Geometry: final body of the model. Coordinates: model frame, mm. A direction names the side the tool comes from. Give positions to 0.01 mm unless a question says otherwise; leave off trailing zeros. Loops run counter-clockwise (first coordinate to the right, second up) from the corner with the lowest first, then second, coordinate; pieces in that order, holes last. Notation, with made-up numbers: (-35, 34) - (-29, 34) arc R19 ccw to (-29, 69) - close; hole circle Ø6 at (55.25, 19). An arc over 180 degrees is marked (long way). Use one line per item in the form item = value.
```python
from build123d import *

# Parameters (mm, degrees)
BASE_FLANGE1_DEPTH = 212.725
FILLET1_R          = 6.35
SKETCH3_R          = 5.5626
SKETCH3_R_2        = 2.1082
CUT_EXTRUDE1_DEPTH = 7.62
CUT_EXTRUDE2_DEPTH = 246.533701925


# Read off the part's stored shape, not the designer's step: Base-Flange1
with BuildPart() as part:
    # Base-Flange1 outline → Base-Flange1 (new body)
    with BuildSketch(Plane.XY):
        with BuildLine():
            Line((-78.007365806, 1.016), (-95.25, 1.016))
            Line((-95.25, 1.016), (-95.25, 0))
            Line((-95.25, 0), (-78.007365806, 0))
            ThreePointArc((-78.007365806, 0), (-76.729452957, 0.520576705), (-76.17906817, 1.7859375))
            ThreePointArc((-76.17906817, 1.7859375), (0, 76.2), (76.17906817, 1.7859375))
            ThreePointArc((76.17906817, 1.7859375), (76.729452957, 0.520576705), (78.007365806, 0))
            Line((78.007365806, 0), (95.25, 0))
            Line((95.25, 0), (95.25, 1.016))
            Line((95.25, 1.016), (78.007365806, 1.016))
            ThreePointArc((78.007365806, 1.016), (77.43940454, 1.247367424), (77.194789079, 1.80975))
            ThreePointArc((77.194789079, 1.80975), (0, 77.216), (-77.194789079, 1.80975))
            ThreePointArc((-77.194789079, 1.80975), (-77.43940454, 1.247367424), (-78.007365806, 1.016))
        make_face()
    extrude(amount=BASE_FLANGE1_DEPTH)

    # Fillet1
    fillet1_edges = [part.edges().sort_by_distance(p)[0] for p in [
        (95.25, 0.508, 0),
        (-95.25, 0.508, 0),
        (95.25, 0.508, 212.725),
        (-95.25, 0.508, 212.725),
    ]]
    fillet(fillet1_edges, radius=FILLET1_R)

    # Sketch3 → Cut-Extrude1 (cut)
    with BuildSketch(Plane.XZ):
        with Locations((-85.725, 9.525)):
            Circle(SKETCH3_R)
        with Locations((-85.725, 25.4)):
            Circle(SKETCH3_R_2)
        with Locations((-85.725, 106.3752)):
            Circle(SKETCH3_R_2)
        with Locations((-85.725, 187.3504)):
            Circle(SKETCH3_R_2)
        with Locations((85.725, 9.525)):
            Circle(SKETCH3_R)
        with Locations((85.725, 25.4)):
            Circle(SKETCH3_R_2)
        with Locations((85.725, 106.3752)):
            Circle(SKETCH3_R_2)
        with Locations((85.725, 187.3504)):
            Circle(SKETCH3_R_2)
    extrude(amount=-CUT_EXTRUDE1_DEPTH, mode=Mode.SUBTRACT)

    # Sketch4 → Cut-Extrude2 (cut, through all)
    with BuildSketch(Plane(origin=(0, 0, 0), x_dir=(0, 0, -1), z_dir=(1, 0, 0))):
        with BuildLine():
            Line((-82.5627, -6.3754), (-82.5627, 9.525))
            ThreePointArc((-82.5627, 9.525), (-74.6125, 17.4752), (-66.6623, 9.525))
            Line((-66.6623, 9.525), (-66.6623, -6.3754))
            Line((-66.6623, -6.3754), (-82.5627, -6.3754))
        make_face()
    extrude(amount=CUT_EXTRUDE2_DEPTH, mode=Mode.SUBTRACT)


solid = part.part
```
(1) Cut plane D-D (x = 0). Return the cut outline in (y, z) (3 decimals), plus the area to 3 significant figures.
Solution:
outline = (76.2, 0) - (77.216, 0) - (77.216, 212.725) - (76.2, 212.725) - close
area = 216 mm2
(2) Pin query (flat end, axial travel): P1, Ø1, axis at x = -20, z = 180.5, coming from the +Y side; P2, Ø7.5, axis at x = 90, y = 7, coming from the -Z side; P3, Ø19, axis at x = 90.5, z = 135.5, coming from the +Y side; P4, Ø3, axis at y = 56.5, z = 132, coming from the +X side. Return the tip coordinate at first contact, or that it passes through.
Solution:
P1 = 74.71
P2 = through
P3 = 1.02
P4 = 54.2
(3) Cut plane A-A (y = 43.5). Return the cut outline in (x, z) (3 decimals), plus the area to 3 significant figures.
Solution:
outline = (-63.797, 0) - (-62.563, 0) - (-62.563, 212.725) - (-63.797, 212.725) - close; (62.563, 0) - (63.797, 0) - (63.797, 212.725) - (62.563, 212.725) - close
area = 525 mm2
(4) Access query for faces 1 (the face through (87, 1.016, 147)), 2 (the face through (91.03, 0.5, 11.2)), 3 (the face through (-88, 1.016, 105)). Directions: +Z, -Z, +X, -X, +Y, -Y. A direction counts if a zero-diameter tool reaches every point of the face in a straight line with its end or side. Return the directions, or none.
Solution:
face_1 = +Z, -Z, +X, +Y
face_2 = +Y, -Y
face_3 = +Z, -Z, -X, +Y
(5) Pull-direction query (Z, two-part tool) for faces 4 (the face through (87, 1.016, 33)), 5 (the face through (74.834, 17.473, 74.787)), 6 (the face through (-93.439, 0.501, 210.815)); classes: released by +Z, released by -Z, zero draft, split by the parting line, or undercut.
Solution:
face_4 = zero draft
face_5 = undercut
face_6 = released by +Z
(6) Material intervals for L1, parallel to X at y = 12.5, z = 161; L2, parallel to X at y = 65, z = 161; L3, parallel to Y at x = -82, z = 126.5, sorted ascending. Write a range as from..to.
Solution:
L1 = -76.2..-75.17, 75.17..76.2
L2 = -41.68..-39.77, 39.77..41.68
L3 = 0..1.02
(7) Cut plane C-C (y = 14). Return the cut outline in (x, z) (3 decimals), plus the area to 3 significant figures.
Solution:
outline = (-75.936, 0) - (-74.903, 0) - (-74.903, 212.725) - (-75.936, 212.725) - close; (74.903, 0) - (75.936, 0) - (75.936, 68.041) - (74.903, 68.041) - close; (74.903, 81.184) - (75.936, 81.184) - (75.936, 212.725) - (74.903, 212.725) - close
area = 426 mm2
